```python
from build123d import *

# Parameters (mm, degrees)
SKETCH1_W           = 15
SKETCH1_H           = 8
BOSS_EXTRUDE2_DEPTH = 18
SKETCH2_W           = 12
SKETCH2_H           = 5
CUT_EXTRUDE1_DEPTH  = 16.5
SKETCH3_W           = 5.25
SKETCH3_H           = 6
CUT_EXTRUDE2_DEPTH  = 8
SKETCH5_W           = 5
SKETCH5_H           = 1.5
CUT_EXTRUDE3_DEPTH  = 15
SKETCH4_W           = 5.25
SKETCH4_H           = 1.5
CUT_EXTRUDE4_DEPTH  = 15
SKETCH6_W           = 15
SKETCH6_H           = 8
CUT_EXTRUDE5_DEPTH  = 1.5


with BuildPart() as part:
    # Sketch1 → Boss-Extrude2 (new body)
    with BuildSketch(Plane(origin=(0, 0, 0), x_dir=(1, 0, 0), z_dir=(0, 1, 0))):
        with Locations((-26.34923581, -20.1983027)):
            Rectangle(SKETCH1_W, SKETCH1_H)
    extrude(amount=BOSS_EXTRUDE2_DEPTH)

    # Sketch2 → Cut-Extrude1 (cut)
    with BuildSketch(Plane(origin=(0, 0, 0), x_dir=(-1, 0, 0), z_dir=(0, -1, 0))):
        with Locations((26.34923581, -20.1983027)):
            Rectangle(SKETCH2_W, SKETCH2_H)
    extrude(amount=-CUT_EXTRUDE1_DEPTH, mode=Mode.SUBTRACT)

    # Sketch3 → Cut-Extrude2 (cut)
    with BuildSketch(Plane.XY.offset(24.1983027)):
        with Locations((-29.72423581, 13.5)):
            Rectangle(SKETCH3_W, SKETCH3_H)
        with Locations((-22.97423581, 13.5)):
            Rectangle(SKETCH3_W, SKETCH3_H)
        with Locations((-22.97423581, 6)):
            Rectangle(SKETCH3_W, SKETCH3_H)
        with Locations((-29.72423581, 6)):
            Rectangle(SKETCH3_W, SKETCH3_H)
    extrude(amount=-CUT_EXTRUDE2_DEPTH, mode=Mode.SUBTRACT)

    # Sketch5 → Cut-Extrude3 (cut)
    with BuildSketch(Plane(origin=(-18.84923581, 0, 0), x_dir=(0, 0, -1), z_dir=(1, 0, 0))):
        with Locations((-20.1983027, 0.75)):
            Rectangle(SKETCH5_W, SKETCH5_H)
    extrude(amount=-CUT_EXTRUDE3_DEPTH, mode=Mode.SUBTRACT)

    # Sketch4 → Cut-Extrude4 (cut)
    with BuildSketch(Plane.XY.offset(24.1983027)):
        with Locations((-29.72423581, 0.75)):
            Rectangle(SKETCH4_W, SKETCH4_H)
        with Locations((-22.97423581, 0.75)):
            Rectangle(SKETCH4_W, SKETCH4_H)
    extrude(amount=-CUT_EXTRUDE4_DEPTH, mode=Mode.SUBTRACT)

    # Sketch6 → Cut-Extrude5 (cut)
    with BuildSketch(Plane.XZ):
        with Locations((-26.34923581, 20.1983027)):
            Rectangle(SKETCH6_W, SKETCH6_H)
    extrude(amount=-CUT_EXTRUDE5_DEPTH, mode=Mode.SUBTRACT)


solid = part.part
```
Check sheet for the modelled part. Datum: model origin and axes. Units: mm. A direction names the side the tool comes from. Coordinates: 2 decimals unless noted, no trailing zeros. Order: outer loops, then holes, each group sorted by start corner. A loop starts at its lowest first (then second) coordinate and runs counter-clockwise, first axis right, second up. Notation, with made-up numbers: M 68,16 L 76,16 A24 cw 76,45 Z; hole C 56.5,8.25 d2. An arc over 180 degrees is marked long. One line per question, with ' | ' between items. Start each with the question number.
Item 1: Material ranges on line 1 (Y direction, x = -28.75, z = 22.75); line 2 (X direction, y = 6.25, z = 17.5); line 3 (X direction, y = 6, z = 18.75), recorded low to high.
Item 2: Gauge pin test, flat end, axial feed: P1, Ø3.5, axis at x = -27.5, y = 8.5, coming from the -Z side. Record the tip position at first contact, or that the pin passes through.
Item 3: Mould release check, pull along Z, two halves, no side actions. Record for faces 1 (the flat face through (-26, 7, 22.698)), 2 (the flat face through (-33.849, 10, 20)), 3 (the flat face through (-26, 10, 24.198)): pulls with the +Z half, pulls with the -Z half, needs draft (parallel to the pull), parting line crosses it, or undercut.
Item 4: Sectioned sample at B-B on y = 3.75. Record the cut outline in (x, z).
Item 5: Access from +Z, -Z, +X, -X, +Y, -Y to the whole of each face (thin tool, end or side, straight path). Record for faces 4 (the flat face through (-26, 1.5, 23)), 5 (the flat face through (-26, 7, 17.698)), 6 (the flat face through (-25.599, 6, 23)).
Item 6: Sectioned sample at A-A on x = -21.75. Record the cut outline in (y, z), and give its area (3 significant figures).
Item 7: Sectioned sample at C-C on z = 17.5. Record the cut outline in (x, y), and give its area (4 significant figures).
Answer below:
1) line 1: y = 1.5 to 3, 9 to 10.5, 16.5 to 18 | line 2: x = -33.85 to -32.35, -27.1 to -25.6, -20.35 to -18.85 | line 3: x = -33.85 to -32.35, -20.35 to -18.85
2) P1: stops at z = 16.2
3) face 1: undercut | face 2: needs draft | face 3: pulls with the +Z half
4) outline: M -33.85,16.2 L -32.35,16.2 L -32.35,24.2 L -33.85,24.2 Z; M -27.1,16.2 L -25.6,16.2 L -25.6,17.7 L -27.1,17.7 Z; M -27.1,22.7 L -25.6,22.7 L -25.6,24.2 L -27.1,24.2 Z; M -20.35,16.2 L -18.85,16.2 L -18.85,24.2 L -20.35,24.2 Z
5) face 4: +Z, -Z, +X, -X, -Y | face 5: -Y | face 6: +Z, -Z
6) outline: M 1.5,16.2 L 3,16.2 L 3,17.7 L 1.5,17.7 Z; M 1.5,22.7 L 3,22.7 L 3,24.2 L 1.5,24.2 Z; M 9,16.2 L 10.5,16.2 L 10.5,17.7 L 9,17.7 Z; M 9,22.7 L 10.5,22.7 L 10.5,24.2 L 9,24.2 Z; M 16.5,16.2 L 18,16.2 L 18,24.2 L 16.5,24.2 Z | area: 21.0 mm^2
7) outline: M -33.85,1.5 L -18.85,1.5 L -18.85,18 L -33.85,18 Z; hole M -32.35,3 L -27.1,3 L -27.1,9 L -32.35,9 Z; hole M -32.35,10.5 L -27.1,10.5 L -27.1,16.5 L -32.35,16.5 Z; hole M -25.6,3 L -20.35,3 L -20.35,9 L -25.6,9 Z; hole M -25.6,10.5 L -20.35,10.5 L -20.35,16.5 L -25.6,16.5 Z | area: 121.5 mm^2
